For this review, take the finished solid that the model builds, in its own axes (mm). A direction names the side the tool comes from. Coordinates: 2 decimals unless noted, no trailing zeros. Loops run counter-clockwise (first coordinate to the right, second up) from the corner with the lowest first, then second, coordinate; pieces in that order, holes last. Notation, with made-up numbers: M 44,-39 L 92,-39 A6 ccw 92,-30 Z; hole C 82,-7.75 d11. An arc over 180 degrees is marked long. Put each result on its own line as item: value.
Autodesk Inventor part; units mm, degrees
ref_plane "YZ Plane" through (0, 0, 0) normal (1, 0, 0) x (0, 1, 0)
ref_plane "XZ Plane" through (0, 0, 0) normal (0, 1, 0) x (-1, 0, 0)
ref_plane "XY Plane" through (0, 0, 0) normal (0, 0, 1) x (1, 0, 0)
sketch "Sketch1" plane through (0, 0, 0) normal (1, 0, 0) x (0, 1, 0)
  arc A0 (0, 32.5) -> (0, 57.5) centre (0, 45) ccw
  arc A1 (0, -57.5) -> (0, -32.5) centre (0, -45) ccw
  line L0 (0, 81.5) -> (17.5, 81.5)
  line L1 (17.5, 81.5) -> (17.5, -81.5)
  line L2 (17.5, -81.5) -> (0, -81.5)
  line L3 (0, 57.5) -> (0, 81.5)
  line L4 (0, -81.5) -> (0, -57.5)
  line L5 (0, -32.5) -> (0, 32.5)
  point P0 (0, 0)
  point P1 (0, 0)
  point P2 (17.5, 0)
  point P3 (0, 69.5)
  point P4 (0, -69.5)
  point P5 (12.5, 45)
  dimension "d0" = 25
  dimension "d2" = 90
  dimension "d3" = 45
  dimension "d4" = 24
  dimension "d15" = 5
extrude "Extrusion1" add sketch "Sketch1" along normal blind 18
sketch "Sketch2" plane through (0, 17.5, 81.5) normal (0, 1, 0) x (1, 0, 0)
  circle A0 centre (9, 9) radius 4.35
  circle A1 centre (9, 154) radius 4.35
  line L0 (18, 163) -> (18, 0)
  line L1 (0, 0) -> (18, 0)
  line L2 (0, 163) -> (18, 163)
  point P0 (0, 81.5)
  dimension "d7" = 8.7
  dimension "d8" = 8.7
  dimension "d9" = 9
  dimension "d10" = 9
  dimension "d11" = 9
extrude "Extrusion2" cut sketch "Sketch2" against normal blind 29.5
sketch "Sketch3" plane through (0, 17.5, 81.5) normal (0, 1, 0) x (1, 0, 0)
  circle A0 centre (9, 154) radius 4.35
  line L0 (12.7528, 160.5) -> (16.5056, 154)
  line L1 (16.5056, 154) -> (12.7528, 147.5)
  line L2 (12.7528, 147.5) -> (5.2472, 147.5)
  line L3 (5.2472, 147.5) -> (1.4944, 154)
  line L4 (1.4944, 154) -> (5.2472, 160.5)
  line L5 (5.2472, 160.5) -> (12.7528, 160.5)
  line L6 (0, 163) -> (18, 163)
  circle A1 centre (9, 9) radius 4.35
  line L7 (12.7528, 2.5) -> (5.2472, 2.5)
  line L8 (5.2472, 2.5) -> (1.4944, 9)
  line L9 (1.4944, 9) -> (5.2472, 15.5)
  line L10 (5.2472, 15.5) -> (12.7528, 15.5)
  line L11 (12.7528, 15.5) -> (16.5056, 9)
  line L12 (16.5056, 9) -> (12.7528, 2.5)
  line L13 (0, 0) -> (18, 0)
  point P0 (0, 81.5)
  dimension "d16" = 13
  dimension "d17" = 13
extrude "Extrusion3" cut sketch "Sketch3" against normal blind 5
sketch "Sketch4" plane through (0, 0, 57.5) normal (0, -1, 0) x (1, 0, 0)
  circle A0 centre (9, 3) radius 1.5
  circle A1 centre (9, -28) radius 1.5
  circle A2 centre (9, -87) radius 1.5
  circle A3 centre (9, -118) radius 1.5
  line L0 (0, 0) -> (18, 0)
  line L1 (0, -25) -> (18, -25)
  line L2 (0, -90) -> (18, -90)
  line L3 (0, -115) -> (18, -115)
  line L4 (0, -139) -> (18, -139)
  point P0 (0, -57.5)
  point P1 (9, -139)
  dimension "d20" = 3
  dimension "d21" = 3
  dimension "d22" = 3
  dimension "d23" = 3
  dimension "d24" = 3
extrude "Extrusion4" cut sketch "Sketch4" against normal blind 22
sketch "Sketch5" plane through (0, 17.5, 81.5) normal (0, 1, 0) x (1, 0, 0)
  circle A0 centre (9, 21) radius 1.5
  line L0 (10.8764, 24.25) -> (12.7528, 21)
  line L1 (12.7528, 21) -> (10.8764, 17.75)
  line L2 (10.8764, 17.75) -> (7.1236, 17.75)
  line L3 (7.1236, 17.75) -> (5.2472, 21)
  line L4 (5.2472, 21) -> (7.1236, 24.25)
  line L5 (7.1236, 24.25) -> (10.8764, 24.25)
  circle A1 centre (9, 52) radius 1.5
  line L6 (7.1236, 55.25) -> (10.8764, 55.25)
  line L7 (10.8764, 55.25) -> (12.7528, 52)
  line L8 (12.7528, 52) -> (10.8764, 48.75)
  line L9 (10.8764, 48.75) -> (7.1236, 48.75)
  line L10 (7.1236, 48.75) -> (5.2472, 52)
  line L11 (5.2472, 52) -> (7.1236, 55.25)
  circle A2 centre (9, 111) radius 1.5
  line L12 (7.1236, 114.25) -> (10.8764, 114.25)
  line L13 (10.8764, 114.25) -> (12.7528, 111)
  line L14 (12.7528, 111) -> (10.8764, 107.75)
  line L15 (10.8764, 107.75) -> (7.1236, 107.75)
  line L16 (7.1236, 107.75) -> (5.2472, 111)
  line L17 (5.2472, 111) -> (7.1236, 114.25)
  circle A3 centre (9, 142) radius 1.5
  line L18 (7.1236, 145.25) -> (10.8764, 145.25)
  line L19 (10.8764, 145.25) -> (12.7528, 142)
  line L20 (12.7528, 142) -> (10.8764, 138.75)
  line L21 (10.8764, 138.75) -> (7.1236, 138.75)
  line L22 (7.1236, 138.75) -> (5.2472, 142)
  line L23 (5.2472, 142) -> (7.1236, 145.25)
  line L24 (12.7528, 147.5) -> (5.2472, 147.5)
  point P0 (0, 81.5)
  dimension "d27" = 6.5
  dimension "d28" = 6.5
  dimension "d29" = 6.5
  dimension "d30" = 6.5
extrude "Extrusion5" cut sketch "Sketch5" against normal blind 7.5
sketch "Sketch6" plane through (18, 0, 0) normal (1, 0, 0) x (0, 0, -1)
  line L0 (-21.25, 13.5) -> (21.25, 13.5)
  line L1 (21.25, 13.5) -> (21.25, 4)
  line L2 (21.25, 4) -> (-21.25, 4)
  line L3 (-21.25, 4) -> (-21.25, 13.5)
  line L4 (-26.25, 17.5) -> (-26.25, 10)
  line L5 (26.25, 17.5) -> (26.25, 10)
  line L6 (81.5, 17.5) -> (-81.5, 17.5)
  point P0 (0, 0)
  dimension "d33" = 5
  dimension "d34" = 5
  dimension "d35" = 4
  dimension "d36" = 4
extrude "Extrusion6" cut sketch "Sketch6" against normal blind 60.25
fillet "Fillet1" radius 2 4 edges at (9, 4, 21.25) (9, 13.5, 21.25) (9, 13.5, -21.25) (9, 4, -21.25)
properties part number "Mount_Block"
(1) Add section D-D (z = 38). Write out the cut boundary in (x, y), plus the area to 3 significant figures.
Determined:
outline: M 0,10.36 L 18,10.36 L 18,17.5 L 0,17.5 Z
area: 129 mm^2
(2) Add section C-C (z = -45). Write out the cut boundary in (x, y).
Determined:
outline: M 0,12.5 L 18,12.5 L 18,17.5 L 0,17.5 Z
(3) Tool access review of faces 4 (the flat face through (11, 10, 60)), 5 (the flat face through (9, 9, 21.25)), 6 (the cylindrical face through (8.874, 12.497, 45.275)): name each direction out of +Z, -Z, +X, -X, +Y, -Y from which nothing blocks a thin tool from reaching the whole face with its end or side.
Determined:
face 4: +Y
face 5: +X, -X
face 6: +X, -X, -Y
(4) Wall thickness on line 1 along Y through (x, z) = (3.25, 3.5); line 2 along X through (y, z) = (7.75, -60.5); line 3 along Z through (x, y) = (1.5, 8.25): over which ranges is each line inside the solid? List them lowest first. Write a range as [from, to].
Determined:
line 1: y = [0, 4], [13.5, 17.5]
line 2: x = [0, 7.5], [10.5, 18]
line 3: z = [-81.5, -54.39], [-35.61, -21.25], [21.25, 35.61], [54.39, 81.5]
(5) Draft analysis for pull direction X (two halves, no side actions). For faces 1 (the flat face through (6.17, 13.8, -62.1)), 2 (the flat face through (11, 10, -61)), 3 (the flat face through (9, 4, 0)), state which applies: +X half, -X half, draft (parallel to the pull), parting line (faces both ways), or undercut.
Determined:
face 1: undercut
face 2: undercut
face 3: draft
(6) Add section A-A (y = 1.75). State how many separate pieces and enclosed holes the cut face has, plus the area to 3 significant figures.
Determined:
separate pieces: 3
enclosed holes: 6
area: 1,900 mm^2
(7) For pin 1 (5 mm diameter, centred on y = 6.5, z = -56.5, fed in from -X), flat-tipped, find the tip position at first contact; note if it passes through.
Determined:
pin 1: stops at x = 0
